Can you work these out from the drawing? Everything is in mm from the part's minimum corner. A direction names the side the tool comes from. Round coordinates to 2 decimals unless told otherwise and drop trailing zeros. Write each loop counter-clockwise with the first axis right and the second up, starting at its lowest first coordinate (ties: lowest second). Pieces come first, ordered by that corner, then holes.
Q1. Please list where these lines run through material, in increasing order: line 1 along X through (y, z) = (2.75, 15.5); line 2 along Z through (x, y) = (6.75, 9.5).
Q2. For the marked faces 4 and 5, which set-ups out of +Z, -Z, +X, -X, +Y, -Y let a thin tool reach every point of the face, with its end or its side?
Q3. If we section it at A-A (z = 15.75): Please give me the cut outline in (x, y), plus the area to 3 significant figures.
Q4. We'd pull the mould along X, two halves only. Please class the marked faces 1, 2 and 3: +X half, -X half, draft (parallel to the pull), parting line (faces both ways), or undercut.
Q5. If we section it at B-B (x = 9.25): Please give me the cut outline in (y, z), plus the area to 3 significant figures.
Q6. I'm going to push a flat-ended pin straight in: pin 1 Ø0.8 at (x, y) = (0.5, 10.5) entering from +Z. Where does the tip first touch, or does it pass through?
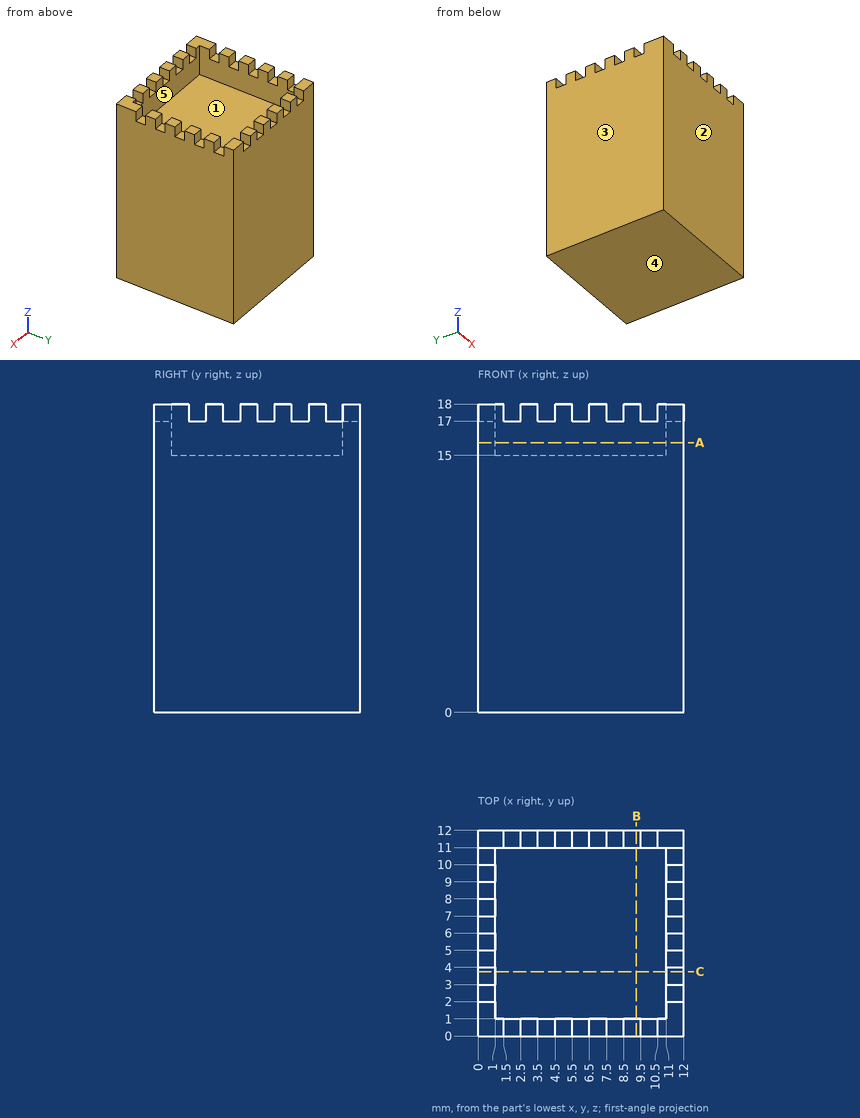
A:
1. line 1: x = 0 to 1, 11 to 12
1. line 2: z = 0 to 15
2. face 4: -Z, +X, -X, +Y, -Y
2. face 5: +Z
3. outline: (0, 0) - (12, 0) - (12, 12) - (0, 12) - close; hole (1, 1) - (11, 1) - (11, 11) - (1, 11) - close
3. area: 44.0 mm2
4. face 1: undercut
4. face 2: draft
4. face 3: -X half
5. outline: (0, 0) - (12, 0) - (12, 18) - (11, 18) - (11, 15) - (1, 15) - (1, 18) - (0, 18) - close
5. area: 186 mm2
6. pin 1: stops at z = 17
